from build123d import *

# Parameters (mm, degrees)
M3X0_5_TAPPED_HOLE1_D      = 2.5
F_10_24_TAPPED_HOLE1_D     = 3.7973
F_10_24_TAPPED_HOLE1_DEPTH = 12.7
F_10_24_TAPPED_HOLE1_TIP   = 1.140824014


with BuildPart() as part:
    # Sketch1 → Revolve1 (revolve)
    with BuildSketch(Plane.XY):
        Polygon((0, 13.8025), (6.5, 13.8025), (6.5, 4.8), (7, 4.8), (7, 2), (11.5, 2), (11.5, 0), (0, 0), align=None)
    revolve(axis=Axis((0, 0, 0), (0, 1, 0)))

    # M3x0.5 Tapped Hole1 (through all)
    with Locations(Plane(origin=(0, 0, 0), x_dir=(-1, 0, 0), z_dir=(0, -1, 0))):
        with Locations((0, 9), (8.559508647, 2.781152949), (5.290067271, -7.281152949), (-5.290067271, -7.281152949), (-8.559508647, 2.781152949), (0, 0)):
            Hole(M3X0_5_TAPPED_HOLE1_D / 2)

    # #10-24 Tapped Hole1
    with Locations(Plane(origin=(0, 13.8025, 0), x_dir=(1, 0, 0), z_dir=(0, 1, 0))):
        with Locations((0, 0)):
            Hole(F_10_24_TAPPED_HOLE1_D / 2, depth=F_10_24_TAPPED_HOLE1_DEPTH)
            with Locations((0, 0, -(F_10_24_TAPPED_HOLE1_DEPTH + F_10_24_TAPPED_HOLE1_TIP / 2))):  # 118° drill point
                Cone(0, F_10_24_TAPPED_HOLE1_D / 2, F_10_24_TAPPED_HOLE1_TIP, mode=Mode.SUBTRACT)


solid = part.part
Can you work these out from the model? Positions are in its coordinate system, mm. A direction names the side the tool comes from. Give positions to 0.01 mm unless a question says otherwise; leave off trailing zeros. Loops run counter-clockwise (first coordinate to the right, second up) from the corner with the lowest first, then second, coordinate; pieces in that order, holes last. Notation, with made-up numbers: (72, 53) -> (88, 53) arc R9 ccw to (88, 58) -> close; hole circle Ø5 at (70.25, 58.25). An arc over 180 degrees is marked (long way). Use one line per item in the form item = value.
1) We'd pull the mould along Z, two halves only. Please class faces 3 (the face through (-5.45, 1.01, 6.04)), 4 (the face through (-1, 13.802, -2)), 5 (the face through (-1.5, 1, -11.4)): released by +Z, released by -Z, zero draft, split by the parting line, or undercut.
Answers:
face_3 = undercut
face_4 = zero draft
face_5 = split by the parting line
2) If we section it at C-C (y = 9): Please give me the cut outline in (x, z), plus the area to 3 significant figures.
Answers:
outline = circle Ø13 at (0, 0); hole circle Ø3.8 at (0, 0)
area = 121 mm²
3) If we section it at D-D (z = -9): Please give me the cut outline in (x, y), plus the area to 3 significant figures.
Answers:
outline = (-7.16, 0) -> (-1.25, 0) -> (-1.25, 2) -> (-7.16, 2) -> close; (1.25, 0) -> (7.16, 0) -> (7.16, 2) -> (1.25, 2) -> close
area = 23.6 mm²
4) If we section it at A-A (x = 0): Please give me the cut outline in (y, z), plus the area to 3 significant figures.
Answers:
outline = (0, -11.5) -> (2, -11.5) -> (2, -10.25) -> (0, -10.25) -> close; (0, -7.75) -> (2, -7.75) -> (2, -7) -> (4.8, -7) -> (4.8, -6.5) -> (13.8, -6.5) -> (13.8, -1.9) -> (1.1, -1.9) -> (0.71, -1.25) -> (0, -1.25) -> close; (0, 1.25) -> (0.71, 1.25) -> (1.1, 1.9) -> (13.8, 1.9) -> (13.8, 6.5) -> (4.8, 6.5) -> (4.8, 7) -> (2, 7) -> (2, 11.5) -> (0, 11.5) -> close
area = 146 mm²
5) I need wall thicknesses on line 1 along Z through (x, y) = (0, 1.5); line 2 along Y through (x, z) = (-9, -0.75); line 3 along Z through (x, y) = (0.5, 2.25). Which ranges of each line are inside material? Lowest first, please.
Answers:
line_1 = -11.5 to -10.25, -7.75 to -1.9, 1.9 to 11.5
line_2 = 0 to 2
line_3 = -6.98 to -1.83, 1.83 to 6.98
6) Will these pins go through, and if not, where does the flat tip stop? pin 1 (1.5 mm diameter, centred on x = 3, y = 6.5, fed in from -Z); pin 2 (4 mm diameter, centred on x = -8, y = 12, fed in from +Z); pin 3 (2 mm diameter, centred on y = 6, z = -9, fed in from -X) (3 decimals); pin 4 (3 mm diameter, centred on x = -8.56, z = -2.78, fed in from +Y).
Answers:
pin_1 = -6.1
pin_2 = 2.5
pin_3 = through
pin_4 = 2
7) If we section it at B-B (z = 0): Please give me the cut outline in (x, y), plus the area to 3 significant figures.
Answers:
outline = (-11.5, 0) -> (-1.25, 0) -> (-1.25, 0.71) -> (-1.9, 1.1) -> (-1.9, 13.8) -> (-6.5, 13.8) -> (-6.5, 4.8) -> (-7, 4.8) -> (-7, 2) -> (-11.5, 2) -> close; (1.25, 0) -> (11.5, 0) -> (11.5, 2) -> (7, 2) -> (7, 4.8) -> (6.5, 4.8) -> (6.5, 13.8) -> (1.9, 13.8) -> (1.9, 1.1) -> (1.25, 0.71) -> close
area = 151 mm²
8) For faces 1 (the face through (9.714, 1.014, -2.302)), 2 (the face through (-1.8, 7.4, -0.6)), which set-ups out of +Z, -Z, +X, -X, +Y, -Y let a thin tool reach every point of the face, with its end or its side?
Answers:
face_1 = +Y, -Y
face_2 = +Y
